Part model, mm, in its own coordinate system. Face numbers are marked on the shaded views. A direction names the side the tool comes from. Round coordinates to 2 decimals unless told otherwise and drop trailing zeros. Loops run counter-clockwise (first coordinate to the right, second up) from the corner with the lowest first, then second, coordinate; pieces in that order, holes last.
1) 3-axis set-ups, long thin cutter, end or side, ignore diameter. For the marked faces 1 and 2: which of +Z, -Z, +X, -X, +Y, -Y reach the whole face in a straight line?
2) Band-saw the part on B-B, the plane x = -46. Write the cut outline in (y, z), then the cut area to 3 significant figures.
3) Band-saw the part on A-A, the plane y = 0. Write the cut outline in (x, z).
4) Band-saw the part on C-C, the plane y = 7. Write the cut outline in (x, z), then the cut area to 3 significant figures.
5) Band-saw the part on D-D, the plane y = -3. Write the cut outline in (x, z).
6) Drop flat-ended pins along their axis: P1, Ø5, axis at y = 13.5, z = -4, coming from the +X side; P2, Ø10, axis at x = 2.5, z = -24, coming from the -Y side; P3, Ø10, axis at x = -29.5, y = 2.5, coming from the -Z side; P4, Ø12, axis at y = 17.5, z = -18.5, coming from the -X side. Give the stop position or say it passes through.
7) Probe line 1 (Y direction, x = -15, z = -25); line 2 (Z direction, x = -38, y = 13). List the from-to ranges inside material, lowest first.
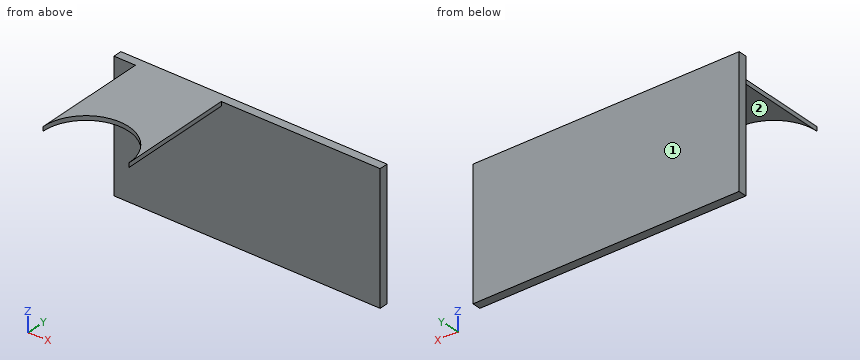
from build123d import *

# Parameters (mm, degrees)
BOSS_EXTRUDE1_DEPTH = 1
BOSS_EXTRUDE2_DEPTH = 2


with BuildPart() as part:
    # Sketch2 → Boss-Extrude1 (new body)
    with BuildSketch(Plane.XY):
        with BuildLine():
            Line((-44.924968499, -5.131156509), (-44.924968499, 21.868843491))
            Line((-44.924968499, 21.868843491), (-24.924968499, 21.868843491))
            Line((-24.924968499, 21.868843491), (-24.924968499, -5.131156509))
            ThreePointArc((-24.924968499, -5.131156509), (-34.924968499, 4.868843491), (-44.924968499, -5.131156509))
        make_face()
    extrude(amount=BOSS_EXTRUDE1_DEPTH)

    # Sketch3 → Boss-Extrude2 (add)
    with BuildSketch(Plane(origin=(0, 21.868843491, 0), x_dir=(1, 0, 0), z_dir=(0, 1, 0))):
        Polygon((-44.924968499, -1), (-49.924968499, -1), (-49.924968499, 29), (12.075031501, 29), (12.075031501, -1), align=None)
    extrude(amount=BOSS_EXTRUDE2_DEPTH)


solid = part.part
Reported:
1. face 1: +Z, -Z, +X, -X, +Y
1. face 2: -Z, +X, -X, -Y
2. outline: (21.87, -29) - (23.87, -29) - (23.87, 1) - (21.87, 1) - close
2. area: 60.0 mm2
3. outline: (-44.92, 0) - (-43.51, 0) - (-43.51, 1) - (-44.92, 1) - close; (-26.34, 0) - (-24.92, 0) - (-24.92, 1) - (-26.34, 1) - close
4. outline: (-44.92, 0) - (-24.92, 0) - (-24.92, 1) - (-44.92, 1) - close
4. area: 20.0 mm2
5. outline: (-44.92, 0) - (-44.7, 0) - (-44.7, 1) - (-44.92, 1) - close; (-25.15, 0) - (-24.92, 0) - (-24.92, 1) - (-25.15, 1) - close
6. P1: passes through
6. P2: stops at y = 21.87
6. P3: stops at z = 0
6. P4: stops at x = -49.92
7. line 1: y = 21.87 to 23.87
7. line 2: z = 0 to 1
